from build123d import *

# Parameters (mm, degrees)
SKETCH1_W           = 90
SKETCH1_H           = 90
SKETCH1_R           = 1.5
SKETCH1_W_2         = 6
SKETCH1_H_2         = 13
BOSS_EXTRUDE9_DEPTH = 5
FILLET2_R           = 10


with BuildPart() as part:
    # Sketch1 → Boss-Extrude9 (new body)
    # profile 1 of 3: a face of its own
    with BuildSketch(Plane(origin=(0, 0, 0), x_dir=(1, 0, 0), z_dir=(0, 1, 0))):
        Polygon((-20, 90), (-20, 60), (0, 0), (0, 90), align=None)
    # profile 2 of 3: a face of its own
    with BuildSketch(Plane(origin=(0, 0, 0), x_dir=(1, 0, 0), z_dir=(0, 1, 0))):
        with Locations((45, 45)):
            Rectangle(SKETCH1_W, SKETCH1_H)
        with Locations(Location((4, 4, 0), (0, 0, 270))):
            Circle(SKETCH1_R, mode=Mode.SUBTRACT)
        with Locations(Location((86, 4, 0), (0, 0, 270))):
            Circle(SKETCH1_R, mode=Mode.SUBTRACT)
        with Locations((5, 75)):
            Rectangle(SKETCH1_W_2, SKETCH1_H_2, mode=Mode.SUBTRACT)
        with Locations(Location((4, 86, 0), (0, 0, 270))):
            Circle(SKETCH1_R, mode=Mode.SUBTRACT)
        with Locations((85, 75)):
            Rectangle(SKETCH1_W_2, SKETCH1_H_2, mode=Mode.SUBTRACT)
        with Locations(Location((86, 86, 0), (0, 0, 270))):
            Circle(SKETCH1_R, mode=Mode.SUBTRACT)
    # profile 3 of 3: a face of its own
    with BuildSketch(Plane(origin=(0, 0, 0), x_dir=(1, 0, 0), z_dir=(0, 1, 0))):
        Polygon((110, 90), (110, 60), (90, 0), (90, 90), align=None)
    extrude(amount=BOSS_EXTRUDE9_DEPTH)

    # Fillet2
    fillet2_edges = [part.edges().sort_by_distance(p)[0] for p in [
        (-20, 2.5, -90),
        (110, 2.5, -90),
        (110, 2.5, -60),
        (90, 2.5, 0),
        (0, 2.5, 0),
        (-20, 2.5, -60),
    ]]
    fillet(fillet2_edges, radius=FILLET2_R)


solid = part.part
Source: CAD feature listing. Evaluate the final solid. Frame: model axes, mm. A direction names the side the tool comes from. Round coordinates to 2 decimals unless told otherwise and drop trailing zeros. Loops run counter-clockwise (first coordinate to the right, second up) from the corner with the lowest first, then second, coordinate; pieces in that order, holes last. Notation, with made-up numbers: M -40,28.25 L -26,28.25 A22 ccw -26,42.25 Z; hole C -37.75,53.5 d1. An arc over 180 degrees is marked long. Answer as CSV lines item,"result".
Q1. Cut plane D-D (z = -4). Return the cut outline in (x, y), plus the area to 3 significant figures.
Verdict:
outline,"M -0.79,0 L 2.5,0 L 2.5,5 L -0.79,5 Z; M 5.5,0 L 84.5,0 L 84.5,5 L 5.5,5 Z; M 87.5,0 L 90.79,0 L 90.79,5 L 87.5,5 Z"
area,"428 mm^2"
Q2. Pull-direction query (X, two-part tool) for faces 3 (the face through (46, 0, -46)), 4 (the face through (85, 2, -81.5)), 5 (the face through (88.57, 2.54, -1.84)); classes: +X half, -X half, draft (parallel to the pull), parting line (faces both ways), or undercut.
Verdict:
face 3,"draft"
face 4,"undercut"
face 5,"+X half"
Q3. Cut plane A-A (z = -72.5). Return the cut outline in (x, y), plus the area to 3 significant figures.
Verdict:
outline,"M -20,0 L 2,0 L 2,5 L -20,5 Z; M 8,0 L 82,0 L 82,5 L 8,5 Z; M 88,0 L 110,0 L 110,5 L 88,5 Z"
area,"590 mm^2"
Q4. Contact query for flat-ended pins moving along their axis: pin 1 (2.5 mm diameter, centred on x = 4, z = -86, fed in from +Y); pin 2 (1.5 mm diameter, centred on x = 85.5, y = 1.5, fed in from +Z); pin 3 (4 mm diameter, centred on x = 86, z = -4, fed in from +Y); pin 4 (1 mm diameter, centred on y = 3.5, z = -18.5, fed in from -X). Output: stop coordinate, or through.
Verdict:
pin 1,"passes through"
pin 2,"stops at z = -0.19"
pin 3,"stops at y = 5"
pin 4,"stops at x = -6.33"
Q5. Cut plane C-C (x = 4). Return the cut outline in (y, z), plus the area to 3 significant figures.
Verdict:
outline,"M 0,-90 L 5,-90 L 5,-87.5 L 0,-87.5 Z; M 0,-84.5 L 5,-84.5 L 5,-81.5 L 0,-81.5 Z; M 0,-68.5 L 5,-68.5 L 5,-5.5 L 0,-5.5 Z; M 0,-2.5 L 5,-2.5 L 5,-0.53 L 0,-0.53 Z"
area,"352 mm^2"
Q6. Line query: line 1 along X through (y, z) = (0.9, -76.5); line 2 along X through (y, z) = (2.4, -86); line 3 along Z through (x, y) = (86, 1.6). Output: solid intervals per line, ascending.
Verdict:
line 1,"x = -20 to 2, 8 to 82, 88 to 110"
line 2,"x = -18 to 2.5, 5.5 to 84.5, 87.5 to 108"
line 3,"z = -90 to -87.5, -84.5 to -81.5, -68.5 to -5.5, -2.5 to -0.53"
Q7. Cut plane B-B (y = 3.2). Return the cut outline in (x, z), plus the area to 3 significant figures.
Verdict:
outline,"M -20,-80 A10 ccw -10,-90 L 100,-90 A10 ccw 110,-80 L 110,-61.62 A10 ccw 109.49,-58.46 L 92.28,-6.84 A10 ccw 82.79,0 L 7.21,0 A10 ccw -2.28,-6.84 L -19.49,-58.46 A10 ccw -20,-61.62 Z; hole M 2,-81.5 L 8,-81.5 L 8,-68.5 L 2,-68.5 Z; hole C 4,-86 d3; hole C 4,-4 d3; hole M 82,-81.5 L 88,-81.5 L 88,-68.5 L 82,-68.5 Z; hole C 86,-86 d3; hole C 86,-4 d3"
area,"10,300 mm^2"
Q8. Reachability of faces 1 (the face through (44, 2, -90)), 2 (the face through (8, 2, -75)) from +Z, -Z, +X, -X, +Y, -Y: full face, straight path, thin tool, end or side. Return the list, or none.
Verdict:
face 1,"-Z, +X, -X, +Y, -Y"
face 2,"+Y, -Y"
